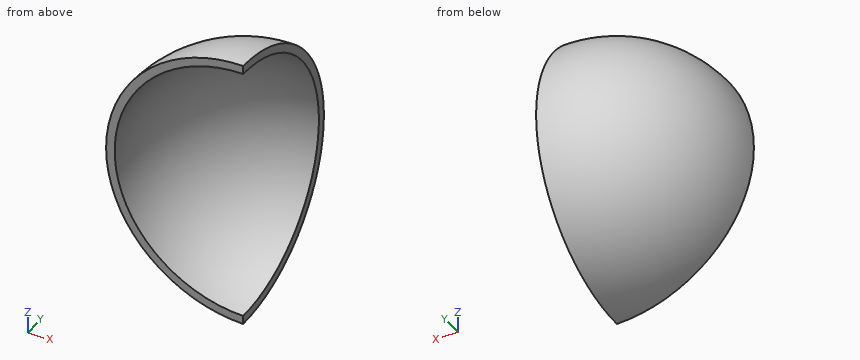
from build123d import *

# Parameters (mm, degrees)
SPHERE001_ANGLE           = 90
SPHERE001_PLACEMENT_ANGLE = 90
SPHERE_ANGLE              = 90
SPHERE_PLACEMENT_ANGLE    = 90


with BuildPart() as sphere001:
    # Sphere001 → Sphere001 (revolve)
    with BuildSketch(Plane.XZ):
        with BuildLine():
            ThreePointArc((0, -750), (750, 0), (0, 750))
            Line((0, 750), (0, -750))
        make_face()
    revolve(axis=Axis((0, 0, 0), (0, 0, 1)), revolution_arc=SPHERE001_ANGLE)


with BuildPart() as sphere001_1:
    # Sphere001 placement: moved
    add(sphere001.part.rotate(Axis((0, 0, 0), (0, 0, 1)), SPHERE001_PLACEMENT_ANGLE))


with BuildPart() as cut:
    # Sphere → Sphere (revolve)
    with BuildSketch(Plane.XZ):
        with BuildLine():
            ThreePointArc((0, -800), (800, 0), (0, 800))
            Line((0, 800), (0, -800))
        make_face()
    revolve(axis=Axis((0, 0, 0), (0, 0, 1)), revolution_arc=SPHERE_ANGLE)


with BuildPart() as cut_1:
    # Sphere placement: moved
    add(cut.part.rotate(Axis((0, 0, 0), (0, 0, 1)), SPHERE_PLACEMENT_ANGLE))

    # Cut: cut Sphere001
    add(sphere001_1.part, mode=Mode.SUBTRACT)


solid = cut_1.part
Geometry: final body of the model. Coordinates: model frame, mm. Give positions to 0.01 mm unless a question says otherwise; leave off trailing zeros. Loops run counter-clockwise (first coordinate to the right, second up) from the corner with the lowest first, then second, coordinate; pieces in that order, holes last. Notation, with made-up numbers: (2, 55) - (30, 55) arc R32 ccw to (30, 89) - close; hole circle Ø8 at (-38, 34). An arc over 180 degrees is marked (long way). Answer as CSV lines item,"result". Start each with the question number.
1. Section B-B, the plane y = 110. Return loops of the section in (x, z).
2. Ray query, L1, parallel to Z at x = -46, y = 531; L2, parallel to Z at x = -433, y = 75.5; L3, parallel to Y at x = -197.5, z = 129. Return the intervals inside material, ascending.
3. Section A-A, the plane z = 482. Return loops of the section in (x, y), plus the area to 3 significant figures.
4. Pin query (flat end, axial travel): P1, Ø12, axis at x = -535, z = -410.5, coming from the -Y side; P2, Ø1, axis at x = -409.5, z = -390.5, coming from the +Y side; P3, Ø4, axis at x = -552, y = 431, coming from the -Z side. Return the tip coordinate at first contact, or that it passes through.
Answers:
1,outline,"(0, -792.4) - (0, -741.89) arc R741.89 cw to (0, 741.89) - (0, 792.4) arc R792.4 ccw to start"
2,L1,"z = -596.59 to -527.66, 527.66 to 596.59"
2,L2,"z = -668.44 to -607.71, 607.71 to 668.44"
2,L3,"y = 711.94 to 764.43"
3,outline,"(-638.5, 0) - (-574.61, 0) arc R574.61 cw to (0, 574.61) - (0, 638.5) arc R638.5 ccw to start"
3,area,"60,900 mm2"
4,P1,"stops at y = 315.65"
4,P2,"stops at y = 566.03"
4,P3,"stops at z = -390.3"
